Source: CAD feature listing. Evaluate the final solid. Frame: model axes, mm. Face numbers are marked on the shaded views. A direction names the side the tool comes from. Round coordinates to 2 decimals unless told otherwise and drop trailing zeros. Order: outer loops, then holes, each group sorted by start corner. A loop starts at its lowest first (then second) coordinate and runs counter-clockwise, first axis right, second up. Notation, with made-up numbers: M 71.5,44 L 97.5,44 A18 ccw 97.5,70 Z; hole C 52.25,77 d11. An arc over 180 degrees is marked long. Answer in a Markdown table with one row per item. Add a question column.
Autodesk Fusion 360 part; units mm, degrees
sketch "Sketch1" plane through (0, 0, 0) normal (0, 0, 1) x (1, 0, 0)
  line L0 (5.65, 0) -> (36.65, 0)
  line L1 (42.3, 5.65) -> (42.3, 36.65)
  line L2 (36.65, 42.3) -> (5.65, 42.3)
  line L3 (0, 36.65) -> (0, 5.65)
  line L4 (42.3, 36.65) -> (36.65, 42.3)
  line L5 (5.65, 42.3) -> (0, 36.65)
  line L6 (36.65, 0) -> (42.3, 5.65)
  line L7 (5.65, 0) -> (0, 5.65)
  dimension "d3" = 5.65
  dimension "d4" = 5.65
  dimension "d9" = 5.65
extrude "Extrude1" add sketch "Sketch1" along normal blind 34
sketch "Sketch2" plane through (0, 0, 34) normal (0, 0, 1) x (-1, 0, 0)
  line L0 (-36.65, 0) -> (-42.3, -5.65)
  line L1 (-42.3, -5.65) -> (-42.3, -36.65)
  line L2 (-42.3, -36.65) -> (-36.65, -42.3)
  line L3 (-36.65, -42.3) -> (-5.65, -42.3)
  line L4 (-5.65, -42.3) -> (0, -36.65)
  line L5 (0, -36.65) -> (0, -5.65)
  line L6 (0, -5.65) -> (-5.65, 0)
  line L7 (-5.65, 0) -> (-36.65, 0)
  circle A0 centre (-21.15, -21.15) radius 11
  circle A1 centre (-5.65, -36.65) radius 1.6
  circle A2 centre (-36.65, -36.65) radius 1.6
  dimension "d12" = 22
  dimension "d13" = 3.2
  dimension "d14" = 3.2
  dimension "d15" = 5.65
  dimension "d16" = 5.65
  dimension "d17" = 5.65
  dimension "d18" = 5.65
  dimension "d19" = 21.15
  dimension "d20" = 21.15
extrude "Extrude3" cut sketch "Sketch2" against normal blind 4.5 contours A1 | A2
extrude "Extrude2" add sketch "Sketch2" along normal blind 2 contours A0
pattern_linear "R-Pattern1" count 2 spacing 31 along (0, -1, 0) of "Extrude3"
sketch "Sketch3" plane through (0, 0, 36) normal (0, 0, 1) x (-1, 0, 0)
  circle A0 centre (-21.15, -21.15) radius 11
  circle A1 centre (-21.15, -21.15) radius 2.5
  dimension "d29" = 5
extrude "Extrude4" add sketch "Sketch3" along normal blind 22 contours A1
sketch "Sketch4" plane through (0, 0, 36) normal (0, 0, 1) x (-1, 0, 0)
  circle A0 centre (-21.15, -21.15) radius 2.5
  circle A1 centre (-21.15, -21.15) radius 11
  circle A2 centre (-21.15, -21.15) radius 4.5
  dimension "d32" = 9
extrude "Extrude5" cut sketch "Sketch4" against normal blind 4.5 contours A2
equation "d3 = ( 11.3 / 2 ) * 1 mm"
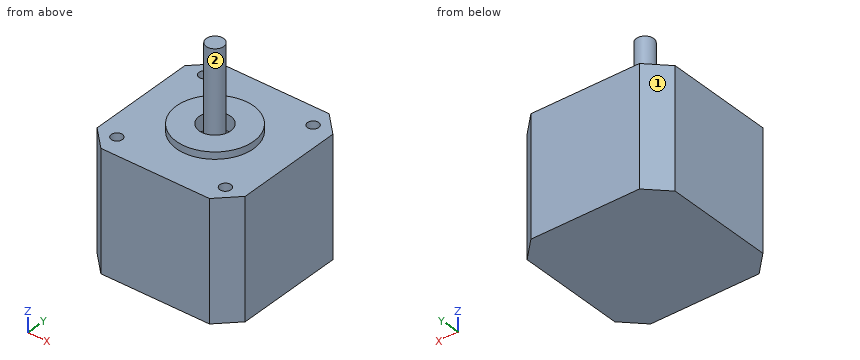
(1) Cut plane D-D (y = 27.5). Return loops of the section in (x, z).
(2) Line query: line 1 (Y direction, x = 36.65, z = 32.9); line 2 (X direction, y = 36, z = 33). Output: solid intervals per line, ascending. Write a range as from..to.
(3) Pin query (flat end, axial travel): pin 1 (2.5 mm diameter, centred on x = 36, y = 6, fed in from +Z); pin 2 (1.6 mm diameter, centred on x = 5.5, y = 6, fed in from +Z); pin 3 (8 mm diameter, centred on x = 6.5, y = 20, fed in from +Z). Return the tip coordinate at first contact, or that it passes through.
(4) Cut plane A-A (z = 4.5). Return loops of the section in (x, y), and give its area (3 significant figures).
(5) Access query for the marked faces 1 and 2. Directions: +Z, -Z, +X, -X, +Y, -Y. A direction counts if a zero-diameter tool reaches every point of the face in a straight line with its end or side. Return the directions, or none.
(6) Cut plane B-B (x = 21.15). Return loops of the section in (y, z), and give its area (3 significant figures).
Answer list:
| question | item | result |
|---|---|---|
| 1 | outline | M 0,0 L 42.3,0 L 42.3,34 L 30.13,34 L 30.13,36 L 12.17,36 L 12.17,34 L 0,34 Z |
| 2 | line 1 | 0..4.05, 7.25..35.05, 38.25..42.3 |
| 2 | line 2 | 0..4.19, 7.11..35.19, 38.11..42.3 |
| 3 | pin 1 | z = 34 |
| 3 | pin 2 | z = 29.5 |
| 3 | pin 3 | z = 36 |
| 4 | outline | M 0,5.65 L 5.65,0 L 36.65,0 L 42.3,5.65 L 42.3,36.65 L 36.65,42.3 L 5.65,42.3 L 0,36.65 Z |
| 4 | area | 1,730 mm² |
| 5 | face 1 | +Z, -Z, -X, +Y |
| 5 | face 2 | +Z |
| 6 | outline | M 0,0 L 42.3,0 L 42.3,34 L 32.15,34 L 32.15,36 L 25.65,36 L 25.65,31.5 L 23.65,31.5 L 23.65,58 L 18.65,58 L 18.65,31.5 L 16.65,31.5 L 16.65,36 L 10.15,36 L 10.15,34 L 0,34 Z |
| 6 | area | 1,570 mm² |
